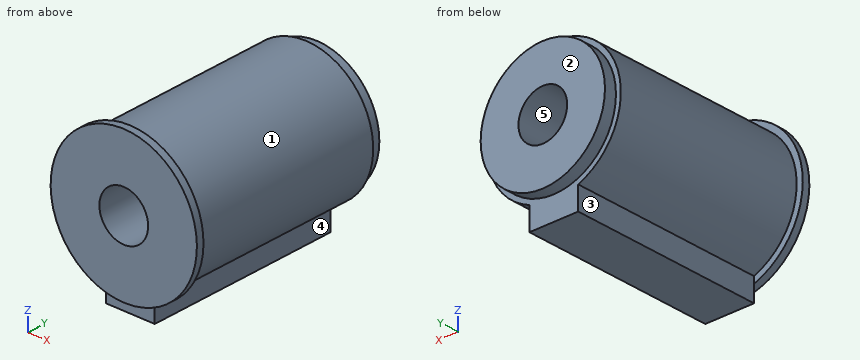
from build123d import *

# Parameters (mm, degrees)
CROQUIS1_R                 = 275
SALIENTE_EXTRUIR1_DEPTH    = 800
SALIENTE_EXTRUIR2_DEPTH    = 800
CROQUIS2_R                 = 300
SALIENTE_EXTRUIR3_DEPTH    = 30
CROQUIS7_R                 = 255
SALIENTE_EXTRUIR4_DEPTH    = 50
CORTAR_EXTRUIR1_DEPTH      = 994.428407083
CORTAR_EXTRUIR1_DEPTH_BACK = 994.428407083
CROQUIS8_R                 = 100


with BuildPart() as part:
    # Croquis1 → Saliente-Extruir1 (new body)
    with BuildSketch(Plane(origin=(0, 0, 0), x_dir=(1, 0, 0), z_dir=(0, 1, 0))):
        with Locations(Location((0, 0, 0), (0, 0, 270))):
            Circle(CROQUIS1_R)
    extrude(amount=SALIENTE_EXTRUIR1_DEPTH)

    # Croquis1_3 → Saliente-Extruir2 (add)
    with BuildSketch(Plane(origin=(0, 0, 0), x_dir=(1, 0, 0), z_dir=(0, 1, 0))):
        with BuildLine():
            Line((0, 350), (-100, 350))
            Line((-100, 350), (-100, 256.173769149))
            ThreePointArc((-100, 256.173769149), (-50.878352391, 270.252462076), (0, 275))
            Line((0, 275), (0, 350))
        make_face()
        with BuildLine():
            Line((100, 350), (0, 350))
            Line((0, 350), (0, 275))
            ThreePointArc((0, 275), (50.878352391, 270.252462076), (100, 256.173769149))
            Line((100, 256.173769149), (100, 350))
        make_face()
    extrude(amount=SALIENTE_EXTRUIR2_DEPTH)

    # Croquis2 → Saliente-Extruir3 (add)
    with BuildSketch(Plane.XZ):
        with Locations(Location((0, 0, 0), (0, 0, 250.528779366))):
            Circle(CROQUIS2_R)
    extrude(amount=SALIENTE_EXTRUIR3_DEPTH)

    # Croquis7 → Saliente-Extruir4 (add)
    with BuildSketch(Plane(origin=(0, 800, 0), x_dir=(1, 0, 0), z_dir=(0, 1, 0))):
        with Locations(Location((0, 0, 0), (0, 0, 270))):
            Circle(CROQUIS7_R)
    extrude(amount=SALIENTE_EXTRUIR4_DEPTH)

    # Croquis8 → Cortar-Extruir1 (cut, two sides: drawn at the far end of the back side and taken through both)
    with BuildSketch(Plane(origin=(0, 850, 0), x_dir=(1, 0, 0), z_dir=(0, 1, 0)).offset(-CORTAR_EXTRUIR1_DEPTH_BACK)):
        with Locations(Location((0, 0, 0), (0, 0, 270))):
            Circle(CROQUIS8_R)
    extrude(amount=CORTAR_EXTRUIR1_DEPTH + CORTAR_EXTRUIR1_DEPTH_BACK, mode=Mode.SUBTRACT)


solid = part.part
Verification items for the finished model (mm, model axes). Face numbers are marked on the shaded views. A direction names the side the tool comes from. Give positions to 0.01 mm unless a question says otherwise; leave off trailing zeros. Loops run counter-clockwise (first coordinate to the right, second up) from the corner with the lowest first, then second, coordinate; pieces in that order, holes last. Notation, with made-up numbers: (73.25, 70.5) - (85.25, 70.5) arc R33 ccw to (85.25, 100.5) - close; hole circle Ø4 at (72, 69.25). An arc over 180 degrees is marked (long way). Write item = value, one per line. Start each with the question number.
Q1. Thickness scan on line 1 (Z direction, x = 0, y = 329); line 2 (X direction, y = 230, z = 0); line 3 (Z direction, x = -66.5, y = 166). Record the ranges inside material, lowest first.
Q2. Cross-section at D-D, the plane x = -168. Enter the section's corners in (y, z).
Q3. Cross-section at A-A, the plane z = 0. Enter the section's corners in (x, y), and give its area (4 significant figures).
Q4. Tool access check on the marked faces 1 and 2. Record the directions out of +Z, -Z, +X, -X, +Y, -Y that give a thin tool (end or side, any length) a straight path to the whole face; none if there is none.
Q5. Cross-section at B-B, the plane x = 0. Enter the section's corners in (y, z).
Q6. Mould release check, pull along X, two halves, no side actions. Record for the marked faces 3, 4 and 5: released by +X, released by -X, zero draft, split by the parting line, or undercut.
Q7. Cross-section at C-C, the plane y = 397. Enter the section's corners in (x, z).
Q8. Depth check by flat-ended pin: P1, Ø1, axis at y = 516.5, z = 234, coming from the -X side; P2, Ø1, axis at x = -54, y = 758, coming from the +Z side. Enter the tip coordinate at first touch or a pass-through.
Answer key:
q1.line_1 = -350 to -100, 100 to 275
q1.line_2 = -275 to -100, 100 to 275
q1.line_3 = -350 to -74.68, 74.68 to 266.84
q2.outline = (-30, -248.55) - (0, -248.55) - (0, -217.72) - (800, -217.72) - (800, -191.84) - (850, -191.84) - (850, 191.84) - (800, 191.84) - (800, 217.72) - (0, 217.72) - (0, 248.55) - (-30, 248.55) - close
q3.outline = (-300, -30) - (-100, -30) - (-100, 850) - (-255, 850) - (-255, 800) - (-275, 800) - (-275, 0) - (-300, 0) - close; (100, -30) - (300, -30) - (300, 0) - (275, 0) - (275, 800) - (255, 800) - (255, 850) - (100, 850) - close
q3.area = 307,500 mm^2
q4.face_1 = +Y
q4.face_2 = +Z, -Z, +X, -X, +Y
q5.outline = (-30, -300) - (0, -300) - (0, -350) - (800, -350) - (800, -255) - (850, -255) - (850, -100) - (-30, -100) - close; (-30, 100) - (850, 100) - (850, 255) - (800, 255) - (800, 275) - (0, 275) - (0, 300) - (-30, 300) - close
q6.face_3 = released by -X
q6.face_4 = released by +X
q6.face_5 = undercut
q7.outline = (-100, -350) - (100, -350) - (100, -256.17) arc R275 ccw (long way) to (-100, -256.17) - close; hole circle Ø200 at (0, 0)
q8.P1 = -145.27
q8.P2 = 269.75
